Can you work these out from the model? Positions are in its coordinate system, mm. Face numbers are marked on the shaded views. Round coordinates to 2 decimals unless told otherwise and drop trailing zeros. Loops run counter-clockwise (first coordinate to the right, second up) from the corner with the lowest first, then second, coordinate; pieces in that order, holes last. Notation, with made-up numbers: (35.25, 84) -> (51.25, 84) arc R25 cw to (51.25, 113) -> close; hole circle Ø6 at (40, 70.25). An arc over 180 degrees is marked (long way). Write item = value, one per line.
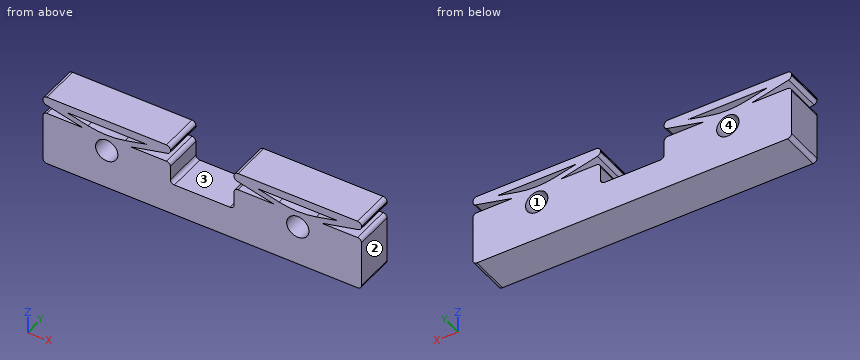
from build123d import *

# Parameters (mm, degrees)
BOSS_EXTRUDE1_DEPTH     = 5
CUT_EXTRUDE1_DEPTH      = 5
CUT_EXTRUDE1_DEPTH_BACK = 10
SKETCH2_R               = 1.4
FILLET1_R               = 10
FILLET2_R               = 0.5


with BuildPart() as part:
    # Sketch1 → Boss-Extrude1 (new body)
    with BuildSketch(Plane(origin=(0, 0, 0), x_dir=(1, 0, 0), z_dir=(0, 1, 0))):
        Polygon((0, 0), (0, 9), (40, 9), (40, 0), (24, 0), (24, 5), (16, 5), (16, 0), align=None)
    extrude(amount=BOSS_EXTRUDE1_DEPTH)

    # Sketch2 → Cut-Extrude1 (cut, two sides: drawn at the far end of the back side and taken through both)
    with BuildSketch(Plane(origin=(0, 5, 0), x_dir=(1, 0, 0), z_dir=(0, 1, 0)).offset(-CUT_EXTRUDE1_DEPTH_BACK)):
        with Locations(Location((8, 4, 0), (0, 0, 270))):
            Circle(SKETCH2_R)
        with Locations(Location((32, 4, 0), (0, 0, 270))):
            Circle(SKETCH2_R)
        Polygon((5, 2.2), (0, 2.2), (0, 1), align=None)
        Polygon((13, 1), (8, 2.2), (3, 1), align=None)
        Polygon((16, 2.2), (11, 2.2), (16, 1), align=None)
        Polygon((24, 2.2), (24, 1), (29, 2.2), align=None)
        Polygon((32, 2.2), (27, 1), (37, 1), align=None)
        Polygon((40, 2.2), (35, 2.2), (40, 1), align=None)
    extrude(amount=CUT_EXTRUDE1_DEPTH + CUT_EXTRUDE1_DEPTH_BACK, mode=Mode.SUBTRACT)

    # Fillet1
    fillet1_edges = [part.edges().sort_by_distance(p)[0] for p in [
        (32, 2.5, -2.2),
        (8, 2.5, -2.2),
    ]]
    fillet(fillet1_edges, radius=FILLET1_R)

    # Fillet2
    fillet2_edges = [part.edges().sort_by_distance(p)[0] for p in [
        (0, 2.5, 0),
        (0, 2.5, -9),
        (40, 2.5, -9),
        (40, 2.5, 0),
        (24, 2.5, 0),
        (24, 2.5, -5),
        (16, 2.5, -5),
        (16, 2.5, 0),
        (0, 2.5, -1),
        (0, 2.5, -2.2),
        (16, 2.5, -2.2),
        (16, 2.5, -1),
        (24, 2.5, -2.2),
        (24, 2.5, -1),
        (40, 2.5, -2.2),
        (40, 2.5, -1),
    ]]
    fillet(fillet2_edges, radius=FILLET2_R)


solid = part.part
1. We'd pull the mould along Z, two halves only. Please class the marked faces 1, 2, 3 and 4: released by +Z, released by -Z, zero draft, split by the parting line, or undercut.
Entries:
face_1 = undercut
face_2 = zero draft
face_3 = released by +Z
face_4 = undercut
2. Suppose I cut it at D-D, the plane y = 3.15. Count the separate pieces of the cut face and the enclosed holes in it, and give its area (3 significant figures).
Entries:
separate_pieces = 1
enclosed_holes = 4
area = 284 mm²
3. I need wall thicknesses on line 1 (X direction, y = 3.45, z = -4); line 2 (Z direction, x = 32, y = 3.65); line 3 (X direction, y = 3.3, z = -5.25). Which ranges of each line are inside material? Lowest first, please. Write a range as [from, to].
Entries:
line_1 = [0, 6.6], [9.4, 16], [24, 30.6], [33.4, 40]
line_2 = [-9, -5.4], [-2.6, -1.92], [-1, 0]
line_3 = [0, 7.37], [8.63, 31.37], [32.63, 40]
4. Suppose I cut it at C-C, the plane x = 26. List the corners of the cut face in (y, z) for me.
Entries:
outline = (0, -9) -> (5, -9) -> (5, -2.2) -> (0, -2.2) -> close; (0, -1.48) -> (5, -1.48) -> (5, 0) -> (0, 0) -> close
5. I'm going to push a flat-ended pin straight in: pin 1 (1.7 mm diameter, centred on x = 8, z = -4, fed in from +Y). Where does the tip first touch, or does it pass through?
Entries:
pin_1 = through
6. Suppose I cut it at B-B, the plane z = -4. List the corners of the cut face in (x, y) for me, and give its area (3 significant figures).
Entries:
outline = (0, 0) -> (6.6, 0) -> (6.6, 5) -> (0, 5) -> close; (9.4, 0) -> (16, 0) -> (16, 5) -> (9.4, 5) -> close; (24, 0) -> (30.6, 0) -> (30.6, 5) -> (24, 5) -> close; (33.4, 0) -> (40, 0) -> (40, 5) -> (33.4, 5) -> close
area = 132 mm²
7. Suppose I cut it at A-A, the plane x = 32. List the corners of the cut face in (y, z) for me.
Entries:
outline = (0, -9) -> (5, -9) -> (5, -5.4) -> (0, -5.4) -> close; (0, -2.6) -> (5, -2.6) -> (5, -1.92) -> (0, -1.92) -> close; (0, -1) -> (5, -1) -> (5, 0) -> (0, 0) -> close
